```python
from build123d import *

# Parameters (mm, degrees)
SKETCH1_R             = 2.625
BOSS_EXTRUDE1_DEPTH   = 2.5
FILLET1_R             = 2.54
M4_CLEARANCE_HOLE1_D  = 4.5
BOSS_EXTRUDE2_DEPTH   = 2.5
BOSS_EXTRUDE2_2_DEPTH = 2.5
FILLET2_R             = 3


with BuildPart() as part:
    # Sketch1 → Boss-Extrude1 (new body)
    # profile 1 of 3: a face of its own
    with BuildSketch(Plane(origin=(0, 0, 0), x_dir=(-1, 0, 0), z_dir=(0, 0, 1))):
        with BuildLine():
            Line((17.121950758, 4.160440607), (32.08303882, 4.160440607))
            Line((32.08303882, 4.160440607), (32.08303882, -8.539559393))
            Line((32.08303882, -8.539559393), (17.121950758, -8.539559393))
            ThreePointArc((17.121950758, -8.539559393), (0.514545783, -19.969559393), (-16.092859192, -8.539559393))
            Line((-16.092859192, -8.539559393), (-31.053947254, -8.539559393))
            Line((-31.053947254, -8.539559393), (-31.053947254, 4.160440607))
            Line((-31.053947254, 4.160440607), (-16.092859192, 4.160440607))
            ThreePointArc((-16.092859192, 4.160440607), (0.514545783, 15.590440607), (17.121950758, 4.160440607))
        make_face()
        with Locations((-23.573403223, -2.189559393)):
            Circle(SKETCH1_R, mode=Mode.SUBTRACT)
        with Locations((24.602494789, -2.189559393)):
            Circle(SKETCH1_R, mode=Mode.SUBTRACT)
    # profile 2 of 3: a face of its own
    with BuildSketch(Plane(origin=(0, 0, 0), x_dir=(-1, 0, 0), z_dir=(0, 0, 1))):
        with Locations((24.602494789, -2.189559393)):
            Circle(SKETCH1_R)
    # profile 3 of 3: a face of its own
    with BuildSketch(Plane(origin=(0, 0, 0), x_dir=(-1, 0, 0), z_dir=(0, 0, 1))):
        with Locations((-23.573403223, -2.189559393)):
            Circle(SKETCH1_R)
    extrude(amount=BOSS_EXTRUDE1_DEPTH)

    # Fillet1
    fillet1_edges = [part.edges().sort_by_distance(p)[0] for p in [
        (-32.08303882, -4.160440607, 1.25),
        (-32.08303882, 8.539559393, 1.25),
        (-17.121950758, 8.539559393, 1.25),
        (16.092859192, 8.539559393, 1.25),
        (31.053947254, 8.539559393, 1.25),
        (31.053947254, -4.160440607, 1.25),
        (16.092859192, -4.160440607, 1.25),
        (-17.121950758, -4.160440607, 1.25),
    ]]
    fillet(fillet1_edges, radius=FILLET1_R)

    # M4 Clearance Hole1 (through all)
    with Locations(Plane.XY.offset(2.5)):
        with Locations((-24.602494789, 2.189559393), (23.573403223, 2.189559393)):
            Hole(M4_CLEARANCE_HOLE1_D / 2)


with BuildPart() as body_2:
    # Sketch4 → Boss-Extrude2 (new body)
    with BuildSketch(Plane.XY.offset(2.5)):
        with BuildLine():
            ThreePointArc((-19.247562091, -4.160440607), (-0.514545783, -17.590440607), (18.218470525, -4.160440607))
            Line((18.218470525, -4.160440607), (17.757572321, -4.160440607))
            ThreePointArc((17.757572321, -4.160440607), (16.410533903, -4.547050837), (15.473557558, -5.589190607))
            ThreePointArc((15.473557558, -5.589190607), (-0.514545783, -15.590440607), (-16.502649124, -5.589190607))
            ThreePointArc((-16.502649124, -5.589190607), (-17.439625469, -4.547050837), (-18.786663887, -4.160440607))
            Line((-18.786663887, -4.160440607), (-19.247562091, -4.160440607))
        make_face()
    extrude(amount=-BOSS_EXTRUDE2_DEPTH)


with BuildPart() as body_3:
    # Sketch4 → Boss-Extrude2 2 (new body)
    with BuildSketch(Plane.XY.offset(2.5)):
        with BuildLine():
            Line((17.757572321, 8.539559393), (18.218470525, 8.539559393))
            ThreePointArc((18.218470525, 8.539559393), (-0.514545783, 21.969559393), (-19.247562091, 8.539559393))
            Line((-19.247562091, 8.539559393), (-18.786663887, 8.539559393))
            ThreePointArc((-18.786663887, 8.539559393), (-17.439625469, 8.926169624), (-16.502649124, 9.968309393))
            ThreePointArc((-16.502649124, 9.968309393), (-0.514545783, 19.969559393), (15.473557558, 9.968309393))
            ThreePointArc((15.473557558, 9.968309393), (16.410533903, 8.926169624), (17.757572321, 8.539559393))
        make_face()
    extrude(amount=-BOSS_EXTRUDE2_2_DEPTH)


with BuildPart() as part_1:
    add(part.part)

    # Combine1: union body 3, body 2
    add(body_3.part)
    add(body_2.part)

    # Fillet2
    fillet2_edges = [part_1.edges().sort_by_distance(p)[0] for p in [
        (-19.247562091, -4.160440607, 1.25),
        (18.218470525, -4.160440607, 1.25),
        (18.218470525, 8.539559393, 1.25),
        (-19.247562091, 8.539559393, 1.25),
    ]]
    fillet(fillet2_edges, radius=FILLET2_R)


solid = part_1.part
```
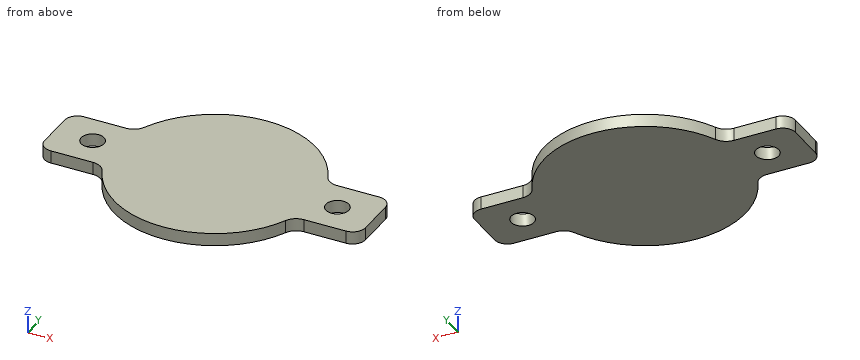
Design review of the part built by this model. Coordinates are the model's own, in mm. Round coordinates to 2 decimals unless told otherwise and drop trailing zeros. Order: outer loops, then holes, each group sorted by start corner. A loop starts at its lowest first (then second) coordinate and runs counter-clockwise, first axis right, second up. Notation, with made-up numbers: M 63.5,86.5 L 82.5,86.5 A15 ccw 82.5,107.5 Z; hole C 64.25,-29.75 d3. An arc over 180 degrees is marked long. Put each result on its own line as item: value.
Q1. Consider section B-B (x = 7). State the section outline as (y, z) points.
Reported:
outline: M -16.11,0 L 20.49,0 L 20.49,2.5 L -16.11,2.5 Z
Q2. Consider section C-C (y = 12). State the section outline as (x, z) points, and give its area (3 significant figures).
Reported:
outline: M -17.69,0 L 16.66,0 L 16.66,2.5 L -17.69,2.5 Z
area: 85.9 mm²
Q3. Insertion check: pin 1 Ø4 at (x, y) = (23.57, 2.19) entering from -Z; pin 2 Ø1.2 at (x, z) = (25.5, 0.5) entering from +Y; pin 3 Ø1.5 at (y, z) = (14.5, 2) entering from +X. Each pin has a flat end and moves straight along its axis. Give the tip position at first contact, or say it passes through.
Reported:
pin 1: through
pin 2: y = 8.54
pin 3: x = 15.54
Q4. To check wall thickness, follow line 1 (X direction, y = 3, z = 0.15); line 2 (Y direction, x = -28, z = 0.2); line 3 (Y direction, x = -1, z = 2.4). State the ranges of each line that lie inside material, in increasing order.
Reported:
line 1: -32.08 to -26.7, -22.5 to 21.47, 25.67 to 31.05
line 2: -4.16 to 8.54
line 3: -17.58 to 21.96
Q5. Consider section A-A (z = 0.6). State the section outline as (x, y) points.
Reported:
outline: M -32.08,-1.62 A2.54 ccw -29.54,-4.16 L -21.29,-4.16 A3 cw -18.55,-5.93 A19.78 ccw 17.52,-5.93 A3 cw 20.26,-4.16 L 28.51,-4.16 A2.54 ccw 31.05,-1.62 L 31.05,6 A2.54 ccw 28.51,8.54 L 20.26,8.54 A3 cw 17.52,10.31 A19.78 ccw -18.55,10.31 A3 cw -21.29,8.54 L -29.54,8.54 A2.54 ccw -32.08,6 Z; hole C -24.6,2.19 d4.5; hole C 23.57,2.19 d4.5
